Could you check a few things on this model? Use its own coordinates, in mm. A direction names the side the tool comes from. Coordinates: 2 decimals unless noted, no trailing zeros. Order: outer loops, then holes, each group sorted by start corner. A loop starts at its lowest first (then second) coordinate and runs counter-clockwise, first axis right, second up. Notation, with made-up numbers: (11.25, 23.5) -> (66.25, 23.5) arc R13 cw to (66.25, 33.5) -> close; hole circle Ø9 at (-32, -2). An arc over 180 degrees is marked (long way). Use a Markdown table: item, result. Add a question column.
1) Which directions (+Z, -Z, +X, -X, +Y, -Y) give clear straight access to the entire face, cutting with the end or side of a thin tool? Please do faces 1 (the flat face through (0, 6, -18)), 2 (the flat face through (-2.4, 3, 2.4)).
2) If we section it at A-A (x = 0): Write out the boundary of the cut face in (y, z).
3) If we section it at D-D (z = 15): Write out the boundary of the cut face in (x, y), plus the area to 3 significant figures.
4) If we section it at C-C (y = 2.25): Write out the boundary of the cut face in (x, z), plus the area to 3 significant figures.
5) Thinking about a two-plate mould opening in Z: for faces 3 (the cylindrical face through (21.07, 3.04, -41)), 4 (the flat face through (22.5, 3, -10)), 5 (the cylindrical face through (-16.474, 2.958, -16.77)), which applies, +Z half, -Z half, draft (parallel to the pull), parting line (faces both ways), or undercut?
6) If we section it at B-B (z = 0): Write out the boundary of the cut face in (x, y).
7) Will these pins go through, and if not, where does the flat tip stop? pin 1 Ø3.5 at (x, z) = (0, 0) entering from +Y; pin 2 Ø6 at (x, z) = (-0.5, 7.5) entering from +Y.
8) If I drill on L1, parallel to X at y = 4, z = -32.5; L2, parallel to X at y = 4.2, z = 0; L3, parallel to Z at x = -15, y = 3.2, over which ranges is the centre line in solid material (lowest first)? Write a range as [from, to].
```python
from build123d import *

# Parameters (mm, degrees)
SKETCH1_W           = 45
SKETCH1_H           = 45
SKETCH1_R           = 3
SKETCH1_R_2         = 1.6
BOSS_EXTRUDE1_DEPTH = 6
SKETCH2_R           = 11.75
CUT_EXTRUDE1_DEPTH  = 3
SKETCH5_W           = 45
SKETCH5_H           = 20
SKETCH5_R           = 2.25
BOSS_EXTRUDE2_DEPTH = 6
FILLET1_R           = 5


with BuildPart() as part:
    # Sketch1 → Boss-Extrude1 (new body)
    with BuildSketch(Plane(origin=(0, 0, 0), x_dir=(1, 0, 0), z_dir=(0, 1, 0))):
        Rectangle(SKETCH1_W, SKETCH1_H)
        with Locations(Location((0, 0, 0), (0, 0, 270))):
            Circle(SKETCH1_R, mode=Mode.SUBTRACT)
        with Locations(Location((-15.50048775, 15.50048775, 0), (0, 0, 270))):
            Circle(SKETCH1_R_2, mode=Mode.SUBTRACT)
        with Locations(Location((15.50048775, 15.50048775, 0), (0, 0, 270))):
            Circle(SKETCH1_R_2, mode=Mode.SUBTRACT)
        with Locations(Location((15.50048775, -15.50048775, 0), (0, 0, 270))):
            Circle(SKETCH1_R_2, mode=Mode.SUBTRACT)
        with Locations(Location((-15.50048775, -15.50048775, 0), (0, 0, 270))):
            Circle(SKETCH1_R_2, mode=Mode.SUBTRACT)
    extrude(amount=BOSS_EXTRUDE1_DEPTH)

    # Sketch2 → Cut-Extrude1 (cut)
    with BuildSketch(Plane(origin=(0, 6, 0), x_dir=(1, 0, 0), z_dir=(0, 1, 0))):
        with Locations(Location((0, 0, 0), (0, 0, 270))):
            Circle(SKETCH2_R)
    extrude(amount=-CUT_EXTRUDE1_DEPTH, mode=Mode.SUBTRACT)

    # Sketch5 → Boss-Extrude2 (add)
    with BuildSketch(Plane(origin=(0, 0, 0), x_dir=(1, 0, 0), z_dir=(0, 1, 0))):
        with Locations((0, 32.5)):
            Rectangle(SKETCH5_W, SKETCH5_H)
        with Locations(Location((-15, 32.5, 0), (0, 0, 90))):
            Circle(SKETCH5_R, mode=Mode.SUBTRACT)
        with Locations(Location((15, 32.5, 0), (0, 0, 90))):
            Circle(SKETCH5_R, mode=Mode.SUBTRACT)
    extrude(amount=BOSS_EXTRUDE2_DEPTH)

    # Fillet1
    fillet1_edges = [part.edges().sort_by_distance(p)[0] for p in [
        (-22.5, 3, -42.5),
        (22.5, 3, -42.5),
        (22.5, 3, 22.5),
        (-22.5, 3, 22.5),
    ]]
    fillet(fillet1_edges, radius=FILLET1_R)


solid = part.part
```
Answer sheet:
| question | item | result |
|---|---|---|
| 1 | face 1 | +Z, -Z, +X, -X, +Y |
| 1 | face 2 | +Y |
| 2 | outline | (0, -42.5) -> (6, -42.5) -> (6, -11.75) -> (3, -11.75) -> (3, -3) -> (0, -3) -> close; (0, 3) -> (3, 3) -> (3, 11.75) -> (6, 11.75) -> (6, 22.5) -> (0, 22.5) -> close |
| 3 | outline | (-22.5, 0) -> (-17.02, 0) -> (-17.02, 6) -> (-22.5, 6) -> close; (-13.98, 0) -> (13.98, 0) -> (13.98, 6) -> (-13.98, 6) -> close; (17.02, 0) -> (22.5, 0) -> (22.5, 6) -> (17.02, 6) -> close |
| 3 | area | 234 mm2 |
| 4 | outline | (-22.5, -37.5) arc R5 ccw to (-17.5, -42.5) -> (17.5, -42.5) arc R5 ccw to (22.5, -37.5) -> (22.5, 17.5) arc R5 ccw to (17.5, 22.5) -> (-17.5, 22.5) arc R5 ccw to (-22.5, 17.5) -> close; hole circle Ø4.5 at (-15, -32.5); hole circle Ø3.2 at (-15.5, -15.5); hole circle Ø3.2 at (-15.5, 15.5); hole circle Ø6 at (0, 0); hole circle Ø4.5 at (15, -32.5); hole circle Ø3.2 at (15.5, -15.5); hole circle Ø3.2 at (15.5, 15.5) |
| 4 | area | 2,810 mm2 |
| 5 | face 3 | -Z half |
| 5 | face 4 | draft |
| 5 | face 5 | undercut |
| 6 | outline | (-22.5, 0) -> (-3, 0) -> (-3, 3) -> (-11.75, 3) -> (-11.75, 6) -> (-22.5, 6) -> close; (3, 0) -> (22.5, 0) -> (22.5, 6) -> (11.75, 6) -> (11.75, 3) -> (3, 3) -> close |
| 7 | pin 1 | through |
| 7 | pin 2 | y = 3 |
| 8 | L1 | [-22.5, -17.25], [-12.75, 12.75], [17.25, 22.5] |
| 8 | L2 | [-22.5, -11.75], [11.75, 22.5] |
| 8 | L3 | [-42.5, -34.75], [-30.25, -17.02], [-13.98, 13.98], [17.02, 22.5] |
